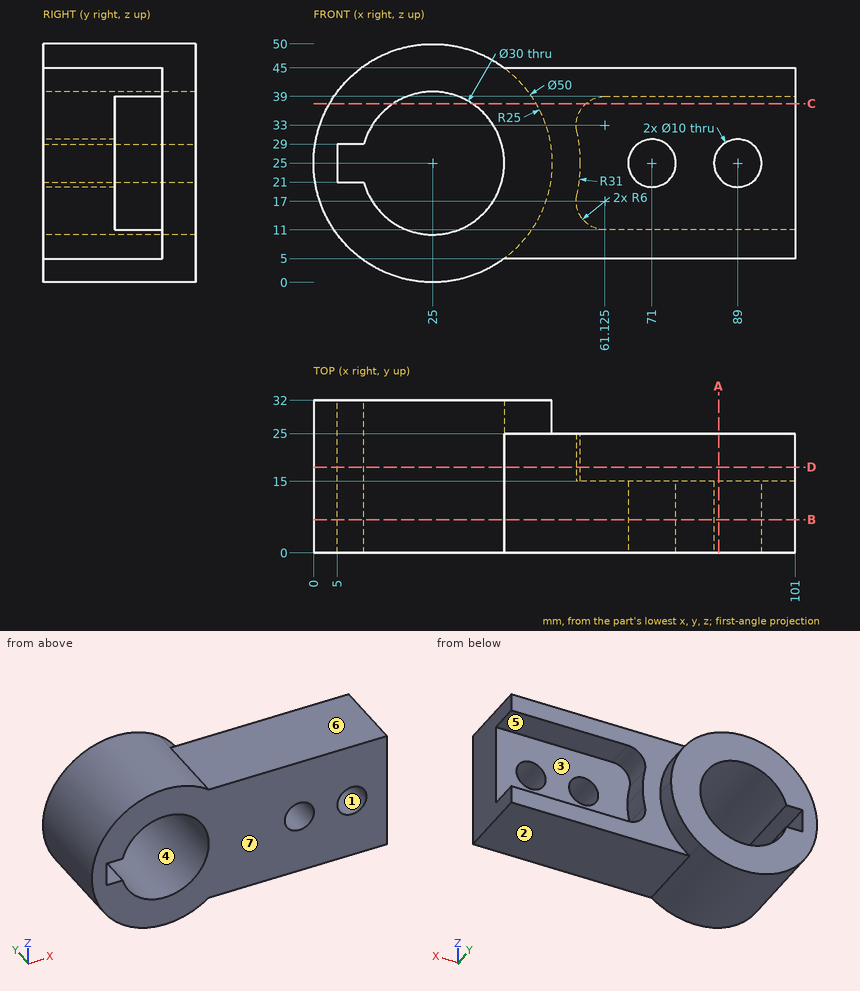
Geometry check sheet. Reference: drawing and pictorial views, mm from the part's lowest x, y, z. A direction names the side the tool comes from. Coordinates: 2 decimals unless noted, no trailing zeros. Order: outer loops, then holes, each group sorted by start corner. A loop starts at its lowest first (then second) coordinate and runs counter-clockwise, first axis right, second up.
Item 1: Tool access check on the marked faces 1, 2 and 3. Record the directions out of +Z, -Z, +X, -X, +Y, -Y that give a thin tool (end or side, any length) a straight path to the whole face; none if there is none.
Item 2: Section check D-D (y = 18). Enter the section's corners in (x, z) (1 decimal).
Item 3: Scan lines: line 1 along Z through (x, y) = (89, 9); line 2 along X through (y, z) = (19, 25); line 3 along Y through (x, z) = (54, 26). Record each from-to range of solid material in increasing order.
Item 4: Depth check by flat-ended pin: pin 1 (3 mm diameter, centred on y = 22.5, z = 33, fed in from +X) (1 decimal); pin 2 (3 mm diameter, centred on x = 71.5, y = 20.5, fed in from -Z); pin 3 (1.5 mm diameter, centred on y = 24.5, z = 27, fed in from -X); pin 4 (6 mm diameter, centred on x = 71, z = 25, fed in from +Y). Enter the tip coordinate at first touch or a pass-through.
Item 5: Section check C-C (z = 37.5). Enter the section's corners in (x, y).
Item 6: Section check A-A (x = 85). Enter the section's corners in (y, z).
Item 7: Section check B-B (y = 7). Enter the section's corners in (x, z).
Item 8: Mould release check, pull along Z, two halves, no side actions. Record for the marked faces 4, 5, 6 and 7: released by +Z, released by -Z, zero draft, split by the parting line, or undercut.
Check sheet entries:
1. face 1: +Y, -Y
1. face 2: -Z, +X, +Y, -Y
1. face 3: +X, +Y
2. outline: (40, 5) - (101, 5) - (101, 11) - (61.1, 11) arc R6 cw to (55.3, 18.3) arc R31 ccw to (55.3, 31.7) arc R6 cw to (61.1, 39) - (101, 39) - (101, 45) - (40, 45) arc R25 ccw (long way) to start; hole (5, 21) - (10.5, 21) arc R15 ccw (long way) to (10.5, 29) - (5, 29) - close
3. line 1: z = 5 to 20, 30 to 45
3. line 2: x = 0 to 5, 40 to 56
3. line 3: y = 0 to 25
4. pin 1: stops at x = 55.3
4. pin 2: stops at z = 5
4. pin 3: stops at x = 0.03
4. pin 4: passes through
5. outline: (3.35, 0) - (16.71, 0) - (16.71, 32) - (3.35, 32) - close; (33.29, 0) - (101, 0) - (101, 15) - (57.16, 15) - (57.16, 25) - (46.65, 25) - (46.65, 32) - (33.29, 32) - close
6. outline: (0, 5) - (25, 5) - (25, 11) - (15, 11) - (15, 22) - (0, 22) - close; (0, 28) - (15, 28) - (15, 39) - (25, 39) - (25, 45) - (0, 45) - close
7. outline: (40, 5) - (101, 5) - (101, 45) - (40, 45) arc R25 ccw (long way) to start; hole (5, 21) - (10.54, 21) arc R15 ccw (long way) to (10.54, 29) - (5, 29) - close; hole circle Ø10 at (71, 25); hole circle Ø10 at (89, 25)
8. face 4: undercut
8. face 5: undercut
8. face 6: released by +Z
8. face 7: zero draft
